from build123d import *

# Parameters (mm, degrees)
F0_W     = 25.4
F0_H     = 2.54
F1_DEPTH = 2.54


with BuildPart() as f1:
    # F0 (on Front) → F1 (new body)
    with BuildSketch(Plane.XZ):
        Polygon((10.900511, 62.895621), (0, 85.837697), (-10.866994, 62.879726), (-21.733987, 39.921754), (-32.600981, 16.963783), (-43.467974, -5.994189), (-54.334968, -28.95216), (-65.201961, -51.910132), (-76.068955, -74.868103), (-50.668955, -74.868103), (-25.268955, -74.868103), (0.131045, -74.868103), (25.531045, -74.868103), (50.931045, -74.868103), (76.356445, -74.868103), (65.455934, -51.926027), (54.555423, -28.983951), (43.654912, -6.041875), (32.7544, 16.900201), (21.801022, 39.953545), align=None)
        Polygon((2.294208, 86.927748), (0, 85.837697), (10.900511, 62.895621), (13.194719, 63.985672), align=None)
        Polygon((-21.733987, 39.921754), (-10.866994, 62.879726), (-13.162791, 63.966425), (-24.029784, 41.008454), align=None)
        Polygon((24.09253, 41.042313), (21.801022, 39.953545), (32.7544, 16.900201), (34.993042, 18.100237), align=None)
        Polygon((-43.467974, -5.994189), (-32.600981, 16.963783), (-34.896778, 18.050482), (-45.763771, -4.907489), align=None)
        Polygon((45.949119, -4.951824), (43.654912, -6.041875), (54.555423, -28.983951), (56.849631, -27.8939), align=None)
        Polygon((-65.201961, -51.910132), (-54.334968, -28.95216), (-56.630765, -27.865461), (-67.497758, -50.823432), align=None)
        Polygon((67.750142, -50.835976), (65.455934, -51.926027), (76.356445, -74.868103), (78.650653, -73.778052), align=None)
        Polygon((76.331045, -77.408103), (76.356445, -74.868103), (50.931045, -74.868103), (50.931045, -77.408103), align=None)
        with Locations((-37.968955, -76.138103)):
            Rectangle(F0_W, F0_H)
        with Locations((12.831045, -76.138103)):
            Rectangle(F0_W, F0_H)
    extrude(amount=F1_DEPTH)


solid = f1.part
Model file for the job. Use its own axes, mm. Give positions to 0.01 mm unless a question says otherwise; leave off trailing zeros. Write each loop counter-clockwise with the first axis right and the second up, starting at its lowest first coordinate (ties: lowest second). Pieces come first, ordered by that corner, then holes. Notation, with made-up numbers: (63.25, -11.75) -> (103.25, -11.75) arc R23 cw to (103.25, 24.25) -> close; hole circle Ø11 at (-1.75, -38). An arc over 180 degrees is marked (long way). Write item = value, one per line.
(1) Mould opens along Z. For faces 1 (the face through (0, 0, -12)), 2 (the face through (7.82, -1.25, 75.3)), 3 (the face through (16.43, -1.25, 51.26)), 4 (the face through (-70.56, -1.25, -63.23)) say: released by +Z, released by -Z, zero draft, split by the parting line, or undercut.
Determined:
face_1 = zero draft
face_2 = released by +Z
face_3 = undercut
face_4 = undercut
(2) Slice it at A-A, the plane z = 71.5. Give the cut face in (x, y).
Determined:
outline = (-6.79, -2.54) -> (9.62, -2.54) -> (9.62, 0) -> (-6.79, 0) -> close
(3) Flat gauge pins, fed straight in: P1, Ø0.8, axis at y = -2, z = -76, coming from the -X side; P2, Ø1.5, axis at y = -1.5, z = 65, coming from the -X side; P3, Ø0.8, axis at x = -57, y = -1, coming from the -Z side. Where does each tip first touch, or does it go through?
Determined:
P1 = -50.67
P2 = -10.22
P3 = -74.87
(4) Probe line 1 along Z through (x, y) = (34, -1.7); line 2 along X through (y, z) = (-2.3, 19.5); line 3 along Z through (x, y) = (-16, -1.15). List the from-to ranges inside material, lowest first.
Determined:
line_1 = -74.87 to 14.28, 17.57 to 20.19
line_2 = -31.4 to 34.33
line_3 = -74.87 to 57.97
(5) Slice it at B-B, the plane x = -61.5. Give the cut face in (y, z), then the cut area to 3 significant figures.
Determined:
outline = (-2.54, -74.87) -> (0, -74.87) -> (0, -38.15) -> (-2.54, -38.15) -> close
area = 93.3 mm2
